Could you check a few things on this model? Use its own coordinates, in mm. A direction names the side the tool comes from. Coordinates: 2 decimals unless noted, no trailing zeros. Loops run counter-clockwise (first coordinate to the right, second up) from the corner with the lowest first, then second, coordinate; pieces in that order, holes last.
1) Imagine slicing it at C-C on x = 20. Please give me the cut outline in (y, z), plus the area to 3 significant figures.
2) Imagine slicing it at D-D on x = 65.5. Please give me the cut outline in (y, z), plus the area to 3 significant figures.
3) Imagine slicing it at B-B on z = 30. Please give me the cut outline in (x, y), plus the area to 3 significant figures.
4) Imagine slicing it at A-A on y = -13. Please give me the cut outline in (x, z).
5) If I drill on line 1 along Z through (x, y) = (20, -15); line 2 along Z through (x, y) = (96, -66.5), over which ranges is the centre line in solid material (lowest first)?
6) Will these pins go through, and if not, where does the flat tip stop? P1, Ø15, axis at x = 18.5, z = -29.5, coming from the -Y side; P2, Ø24, axis at x = 83, y = -68.5, coming from the -Z side; P3, Ø12, axis at y = -102.5, z = -19, coming from the -X side.
7) For faces 4 (the face through (106.925, -89, -12)), 5 (the face through (50, -12, 22)), 6 (the face through (66, -88, -25)), 7 (the face through (29, -31, -50)), 8 (the face through (36, -25, 25)), which set-ups out of +Z, -Z, +X, -X, +Y, -Y let a thin tool reach every point of the face, with its end or its side?
8) Thinking about a two-plate mould opening in X: for faces 1 (the face through (83, -43.267, -12)), 2 (the face through (8.944, -12.675, 40.138)), 3 (the face through (26.762, -97, -12)), which applies, released by +X, released by -X, zero draft, split by the parting line, or undercut?
```python
from build123d import *

# Parameters (mm, degrees)
F0_W       = 50
F0_H       = 50
F1_DEPTH   = 25
F2_R       = 5
F3_R       = 15
F4_DEPTH   = 25.001
F5_W       = 59.2767745256
F5_H       = 61.2553304527
F6_DEPTH   = 25
F6_FACE1_W = 59.2767745256
F6_FACE1_H = 61.2553304527
F7_W       = 7.189117372
F7_H       = 74.1506516933
F8_DEPTH   = 25


with BuildPart() as f1:
    # F0 (on Front) → F1 (new body)
    with BuildSketch(Plane.XZ):
        with Locations((25, 25)):
            Rectangle(F0_W, F0_H)
    extrude(amount=F1_DEPTH)

    # F2
    f2_edges = [f1.edges().sort_by_distance(p)[0] for p in [
        (50, -12.5, 50),
    ]]
    fillet(f2_edges, radius=F2_R)

    # F3 (on face) → F4 (cut, through all)
    with BuildSketch(Plane.XZ.offset(25)):
        with Locations((20, 30)):
            Circle(F3_R)
    extrude(amount=-F4_DEPTH, mode=Mode.SUBTRACT)

    # F5 (on Top) → F6 (join)
    with BuildSketch(Plane.XY):
        with Locations((29.6383872628, -30.6276652263)):
            Rectangle(F5_W, F5_H)
    extrude(amount=-F6_DEPTH)

    # F6_face1 (on face) + F7 (on face) → F8 (join)
    with BuildSketch(Plane(origin=(29.6383872628, -30.6276652263, -25), x_dir=(1, 0, 0), z_dir=(0, 0, -1))):
        Rectangle(F6_FACE1_W, F6_FACE1_H)
    with BuildSketch(Plane.XY):
        Polygon((59.2767745256, -61.2553304527), (38.7707948685, -61.2553304527), (36.2086445093, -61.2553304527), (26.7624184489, -61.2553304527), (26.7624184489, -133.4375590086), (106.9246456027, -133.4375590086), (106.9246456027, -43.2669967413), (59.2767745256, -43.2669967413), align=None)
        with Locations((79.3372057378, -86.4168554544)):
            Rectangle(F7_W, F7_H, mode=Mode.SUBTRACT)
        with Locations((79.3372057378, -86.4168554544)):
            Rectangle(F7_W, F7_H)
    extrude(amount=F8_DEPTH, dir=(0, 0, -1))


solid = f1.part
```
Filled in:
1. outline: (-61.26, -50) - (0, -50) - (0, 15) - (-25, 15) - (-25, 0) - (-61.26, 0) - close; (-25, 45) - (0, 45) - (0, 50) - (-25, 50) - close
1. area: 3,560 mm2
2. outline: (-133.44, -25) - (-43.27, -25) - (-43.27, 0) - (-133.44, 0) - close
2. area: 2,250 mm2
3. outline: (0, -25) - (5, -25) - (5, 0) - (0, 0) - close; (35, -25) - (50, -25) - (50, 0) - (35, 0) - close
3. area: 500 mm2
4. outline: (0, -50) - (59.28, -50) - (59.28, 0) - (50, 0) - (50, 45) arc R5 ccw to (45, 50) - (0, 50) - close; hole circle Ø30 at (20, 30)
5. line 1: z = -50 to 15, 45 to 50
5. line 2: z = -25 to 0
6. P1: stops at y = -61.26
6. P2: stops at z = -25
6. P3: stops at x = 26.76
7. face 4: +Z, -Z, +X, +Y, -Y
7. face 5: +Z, +X, +Y, -Y
7. face 6: -Z, +X, -Y
7. face 7: -Z, +X, -X, +Y, -Y
7. face 8: +Z, +X, -X, -Y
8. face 1: zero draft
8. face 2: undercut
8. face 3: released by -X
